The model under review builds one solid part; all positions refer to its coordinate system, in mm. Face numbers are marked on the shaded views. A direction names the side the tool comes from. Round coordinates to 2 decimals unless told otherwise and drop trailing zeros. Write each loop counter-clockwise with the first axis right and the second up, starting at its lowest first coordinate (ties: lowest second). Pieces come first, ordered by that corner, then holes. Notation, with made-up numbers: (5, -12.75) -> (40, -12.75) arc R27 ccw to (40, 20.25) -> close; hole circle Ø1 at (20, 74.25). An arc over 180 degrees is marked (long way). Answer as a JSON object with one key per item and string values. Group by question number.
1) We need section A-A, the plane y = 7.75. Write out the cut boundary in (x, z), then the cut area to 3 significant figures.
2) Insertion check: pin 1 Ø3 at (x, y) = (-8, 8) entering from +Z. The pin has a flat end and moves straight along its axis. Give the tip position at first contact, or say it passes through.
3) We need section D-D, the plane y = 2. Write out the cut boundary in (x, z), then the cut area to 3 significant figures.
4) We need section C-C, the plane x = -15.25. Write out the cut boundary in (y, z), then the cut area to 3 significant figures.
5) Machinability: for the marked faces 1, 2 and 3, which of the approach directions +Z, -Z, +X, -X, +Y, -Y give a long, thin tool a straight path to every point of the face, cutting with its end or side? Answer none if there is none.
6) Mouldability with a two-part tool opening along Z and no side actions: class the marked faces 4, 5, 6 and 7 as pulls with the +Z half, pulls with the -Z half, needs draft (parallel to the pull), parting line crosses it, or undercut.
7) To check wall thickness, follow probe 1 along Y at (x, z) = (-16, 3.5); probe 2 along Y at (x, z) = (-15.25, -2.5); probe 3 along Z at (x, y) = (0, 8.5). State the ranges of each line that lie inside material, in increasing order. Write a range as [from, to].
8) We need section B-B, the plane z = 0. Write out the cut boundary in (x, y), then the cut area to 3 significant figures.
from build123d import *

# Parameters (mm, degrees)
SKETCH1_W           = 30
SKETCH1_H           = 13
BOSS_EXTRUDE1_DEPTH = 15.5
CUT_EXTRUDE1_DEPTH  = 35.933544052
SKETCH3_R           = 1.75
CUT_EXTRUDE2_DEPTH  = 28.753378173


with BuildPart() as part:
    # Sketch1 → Boss-Extrude1 (new body)
    with BuildSketch(Plane(origin=(0, 0, 0), x_dir=(1, 0, 0), z_dir=(0, 1, 0))):
        with Locations((-4, -2.45)):
            Rectangle(SKETCH1_W, SKETCH1_H)
        with BuildLine():
            Line((-1.224744871, -0.95), (1.224744871, -0.95))
            ThreePointArc((1.224744871, -0.95), (0, 1.55), (-1.224744871, -0.95))
        make_face(mode=Mode.SUBTRACT)
    extrude(amount=BOSS_EXTRUDE1_DEPTH)

    # Sketch2 → Cut-Extrude1 (cut, through all)
    with BuildSketch(Plane.ZY.offset(19)):
        Polygon((8.95, 12.25), (6.45, 12.25), (6.45, 13), (3.45, 13), (3.45, 2.5), (6.45, 2.5), (6.45, 3.25), (8.95, 3.25), align=None)
    extrude(amount=-CUT_EXTRUDE1_DEPTH, mode=Mode.SUBTRACT)

    # Sketch3 → Cut-Extrude2 (cut, through all)
    with BuildSketch(Plane(origin=(0, 0, -4.05), x_dir=(-1, 0, 0), z_dir=(0, 0, -1))):
        with Locations((15.25, 7.75)):
            Circle(SKETCH3_R)
    extrude(amount=-CUT_EXTRUDE2_DEPTH, mode=Mode.SUBTRACT)


solid = part.part
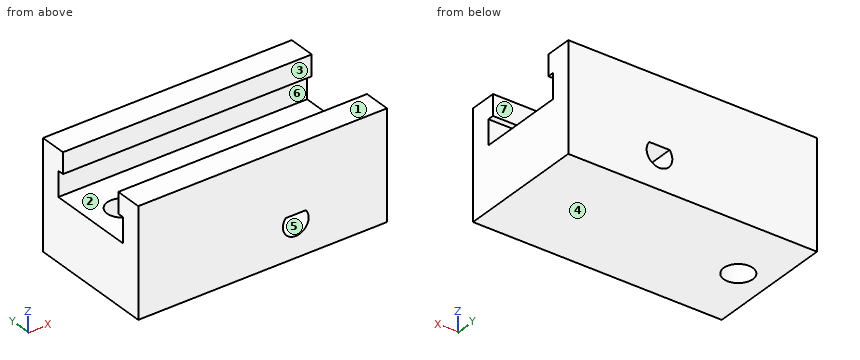
Here are the results:
{
 "1": {"outline": "(-19, -4.05) -> (-17, -4.05) -> (-17, 3.45) -> (-19, 3.45) -> close; (-13.5, -4.05) -> (11, -4.05) -> (11, 3.45) -> (-13.5, 3.45) -> close; hole (-1.22, 0.95) arc R1.55 ccw (long way) to (1.22, 0.95) -> close", "area": "192 mm^2"},
 "2": {"pin 1": "stops at z = 3.45"},
 "3": {"outline": "(-19, -4.05) -> (11, -4.05) -> (11, 8.95) -> (-19, 8.95) -> close; hole (-1.22, 0.95) arc R1.55 ccw (long way) to (1.22, 0.95) -> close", "area": "383 mm^2"},
 "4": {"outline": "(0, -4.05) -> (6, -4.05) -> (6, 3.45) -> (2.5, 3.45) -> (2.5, 6.45) -> (3.25, 6.45) -> (3.25, 8.95) -> (0, 8.95) -> close; (9.5, -4.05) -> (15.5, -4.05) -> (15.5, 8.95) -> (12.25, 8.95) -> (12.25, 6.45) -> (13, 6.45) -> (13, 3.45) -> (9.5, 3.45) -> close", "area": "121 mm^2"},
 "5": {"face 1": "+Z, +X, -X, +Y, -Y", "face 2": "+X, -X", "face 3": "+Z, +X, -X"},
 "6": {"face 4": "pulls with the -Z half", "face 5": "undercut", "face 6": "undercut", "face 7": "needs draft"},
 "7": {"probe 1": "y = [0, 2.5], [13, 15.5]", "probe 2": "y = [0, 6], [9.5, 15.5]", "probe 3": "z = [-4.05, -1.55], [0.95, 3.45]"},
 "8": {"outline": "(-19, 0) -> (-1.55, 0) -> (-1.55, 15.5) -> (-19, 15.5) -> close; (1.55, 0) -> (11, 0) -> (11, 15.5) -> (1.55, 15.5) -> close; hole circle Ø3.5 at (-15.25, 7.75)", "area": "407 mm^2"}
}
